Model file for the job. Use its own axes, mm. A direction names the side the tool comes from. Coordinates: 2 decimals unless noted, no trailing zeros. Loops run counter-clockwise (first coordinate to the right, second up) from the corner with the lowest first, then second, coordinate; pieces in that order, holes last.
from build123d import *

# Parameters (mm, degrees)
SKETCH1_W               = 130
SKETCH1_H               = 80
BOSS_EXTRUDE1_DEPTH     = 5
SKETCH2_W               = 10
SKETCH2_H               = 80
BOSS_EXTRUDE2_DEPTH     = 45
SKETCH3_R               = 1.375
CUT_EXTRUDE1_DEPTH      = 46
CUT_EXTRUDE1_DEPTH_BACK = 6
BOSS_EXTRUDE3_DEPTH     = 10
BOSS_EXTRUDE4_DEPTH     = 10


with BuildPart() as part:
    # Sketch1 → Boss-Extrude1 (new body)
    with BuildSketch(Plane(origin=(0, 0, 0), x_dir=(1, 0, 0), z_dir=(0, 1, 0))):
        Rectangle(SKETCH1_W, SKETCH1_H)
    extrude(amount=BOSS_EXTRUDE1_DEPTH)

    # Sketch2 → Boss-Extrude2 (add)
    with BuildSketch(Plane(origin=(0, 5, 0), x_dir=(1, 0, 0), z_dir=(0, 1, 0))):
        with Locations((60, 0)):
            Rectangle(SKETCH2_W, SKETCH2_H)
        with Locations((-60, 0)):
            Rectangle(SKETCH2_W, SKETCH2_H)
    extrude(amount=BOSS_EXTRUDE2_DEPTH)

    # Sketch3 → Cut-Extrude1 (cut, two sides)
    with BuildSketch(Plane(origin=(0, 5, 0), x_dir=(1, 0, 0), z_dir=(0, 1, 0))) as cut_extrude1_sk:
        with Locations((-46, -22)):
            Circle(SKETCH3_R)
        with Locations((40, -22)):
            Circle(SKETCH3_R)
        with Locations((40, 36)):
            Circle(SKETCH3_R)
        with Locations((-46, 36)):
            Circle(SKETCH3_R)
    extrude(amount=CUT_EXTRUDE1_DEPTH, mode=Mode.SUBTRACT)
    extrude(cut_extrude1_sk.sketch, amount=-CUT_EXTRUDE1_DEPTH_BACK, mode=Mode.SUBTRACT)

    # Sketch4 → Boss-Extrude3 (add)
    with BuildSketch(Plane.ZY.offset(65)):
        with BuildLine():
            Line((-80, 50), (-70, 50))
            ThreePointArc((-70, 50), (-60, 60), (-50, 50))
            Line((-50, 50), (-40, 50))
            ThreePointArc((-40, 50), (-60, 70), (-80, 50))
        make_face()
        with BuildLine():
            Line((-40, 50), (-50, 50))
            ThreePointArc((-50, 50), (-47.071067812, 42.928932188), (-40, 40))
            Line((-40, 40), (-40, 50))
        make_face()
        with BuildLine():
            ThreePointArc((50, 50), (60, 60), (70, 50))
            Line((70, 50), (80, 50))
            ThreePointArc((80, 50), (60, 70), (40, 50))
            Line((40, 50), (50, 50))
        make_face()
        with BuildLine():
            ThreePointArc((40, 40), (47.071067812, 42.928932188), (50, 50))
            Line((50, 50), (40, 50))
            Line((40, 50), (40, 40))
        make_face()
    extrude(amount=-BOSS_EXTRUDE3_DEPTH)

    # Sketch5 → Boss-Extrude4 (add)
    with BuildSketch(Plane(origin=(65, 0, 0), x_dir=(0, 0, -1), z_dir=(1, 0, 0))):
        with BuildLine():
            ThreePointArc((-50, 50), (-47.071067812, 42.928932188), (-40, 40))
            Line((-40, 40), (-40, 50))
            ThreePointArc((-40, 50), (-60, 70), (-80, 50))
            Line((-80, 50), (-70, 50))
            ThreePointArc((-70, 50), (-60, 60), (-50, 50))
        make_face()
        with BuildLine():
            Line((40, 50), (40, 40))
            ThreePointArc((40, 40), (47.071067812, 42.928932188), (50, 50))
            ThreePointArc((50, 50), (60, 60), (70, 50))
            Line((70, 50), (80, 50))
            ThreePointArc((80, 50), (60, 70), (40, 50))
        make_face()
    extrude(amount=-BOSS_EXTRUDE4_DEPTH)


solid = part.part
Q1. Slice it at A-A (z = 60). List the corners of the cut face in (x, y), and give its area (3 significant figures).
Answers:
outline: (-65, 60) - (-55, 60) - (-55, 70) - (-65, 70) - close; (55, 60) - (65, 60) - (65, 70) - (55, 70) - close
area: 200 mm2
Q2. Flat gauge pins, fed straight in: P1, Ø8, axis at x = 61, z = -6, coming from the +Y side; P2, Ø20, axis at x = 3.5, y = 22, coming from the +Z side; P3, Ø3, axis at x = -46, z = 22, coming from the +Y side; P4, Ø5, axis at x = -58.5, z = -73.5, coming from the -Y side. Where does each tip first touch, or does it go through?
Answers:
P1: stops at y = 50
P2: passes through
P3: stops at y = 5
P4: stops at y = 50
Q3. Which spindle directions (+Z, -Z, +X, -X, +Y, -Y) get a long thin tool onto all of the face, cutting with end or side? Do faces 4 (the flat face through (-60, 50, -75)), 5 (the flat face through (60, 50, 75)), 6 (the flat face through (55, 38, 1)). Say none if no direction does.
Answers:
face 4: -Z, +X, -X, -Y
face 5: +Z, +X, -X, -Y
face 6: +Z, -Z, +Y
Q4. Mould opens along X. For faces 1 (the flat face through (-55, 38, -1)), 2 (the cylindrical face through (60, 70, -60)), 3 (the flat face through (65, 35, 1)) say: +X half, -X half, draft (parallel to the pull), parting line (faces both ways), or undercut.
Answers:
face 1: undercut
face 2: draft
face 3: +X half
Q5. Slice it at D-D (z = 2). List the corners of the cut face in (x, y).
Answers:
outline: (-65, 0) - (65, 0) - (65, 50) - (55, 50) - (55, 5) - (-55, 5) - (-55, 50) - (-65, 50) - close
Q6. Slice it at C-C (y = 52.5). Count the separate pieces of the cut face and the enclosed holes in it, and give its area (3 significant figures).
Answers:
separate pieces: 8
enclosed holes: 0
area: 813 mm2
Q7. Drill centre lines: line 1 (Z direction, x = 40, y = 2.1) (3 decimals); line 2 (X direction, y = 2, z = 22) (3 decimals); line 3 (X direction, y = 27, z = -5). Where is each one in solid material? Low to high.
Answers:
line 1: z = -40 to -37.375, -34.625 to 20.625, 23.375 to 40
line 2: x = -65 to -47.375, -44.625 to 38.625, 41.375 to 65
line 3: x = -65 to -55, 55 to 65
Q8. Slice it at B-B (y = 42). List the corners of the cut face in (x, z).
Answers:
outline: (-65, -46) - (-55, -46) - (-55, 46) - (-65, 46) - close; (55, -46) - (65, -46) - (65, 46) - (55, 46) - close
